```python
from build123d import *

# Parameters (mm, degrees)
BOSS_EXTRUDE1_DEPTH = 4
SKETCH2_W           = 92
SKETCH2_H           = 107
BOSS_EXTRUDE2_DEPTH = 13.5
SKETCH3_W           = 84
SKETCH3_H           = 27.9
BOSS_EXTRUDE3_DEPTH = 15
SKETCH4_W           = 79
SKETCH4_H           = 9
CUT_EXTRUDE1_DEPTH  = 89.324685111
SKETCH5_W           = 54
SKETCH5_H           = 8
CUT_EXTRUDE2_DEPTH  = 1
BOSS_EXTRUDE4_DEPTH = 17


with BuildPart() as part:
    # Sketch1 → Boss-Extrude1 (new body)
    with BuildSketch(Plane.XY):
        with BuildLine():
            Line((22.5, 58.5), (22.5, 67))
            Line((22.5, 67), (-22.5, 67))
            Line((-22.5, 67), (-22.5, 58.5))
            ThreePointArc((-22.5, 58.5), (-25.5, 55.5), (-28.5, 58.5))
            Line((-28.5, 58.5), (-28.5, 67))
            Line((-28.5, 67), (-50, 67))
            Line((-50, 67), (-50, 61.5))
            Line((-50, 61.5), (-42, 61.5))
            ThreePointArc((-42, 61.5), (-39, 58.5), (-42, 55.5))
            Line((-42, 55.5), (-50, 55.5))
            Line((-50, 55.5), (-50, -55.5))
            Line((-50, -55.5), (-42, -55.5))
            ThreePointArc((-42, -55.5), (-39, -58.5), (-42, -61.5))
            Line((-42, -61.5), (-50, -61.5))
            Line((-50, -61.5), (-50, -67))
            Line((-50, -67), (-28.5, -67))
            Line((-28.5, -67), (-28.5, -58.5))
            ThreePointArc((-28.5, -58.5), (-25.5, -55.5), (-22.5, -58.5))
            Line((-22.5, -58.5), (-22.5, -67))
            Line((-22.5, -67), (22.5, -67))
            Line((22.5, -67), (22.5, -58.5))
            ThreePointArc((22.5, -58.5), (25.5, -55.5), (28.5, -58.5))
            Line((28.5, -58.5), (28.5, -67))
            Line((28.5, -67), (50, -67))
            Line((50, -67), (50, -61.5))
            Line((50, -61.5), (42, -61.5))
            ThreePointArc((42, -61.5), (39, -58.5), (42, -55.5))
            Line((42, -55.5), (50, -55.5))
            Line((50, -55.5), (50, 55.5))
            Line((50, 55.5), (42, 55.5))
            ThreePointArc((42, 55.5), (39, 58.5), (42, 61.5))
            Line((42, 61.5), (50, 61.5))
            Line((50, 61.5), (50, 67))
            Line((50, 67), (28.5, 67))
            Line((28.5, 67), (28.5, 58.5))
            ThreePointArc((28.5, 58.5), (25.5, 55.5), (22.5, 58.5))
        make_face()
    extrude(amount=BOSS_EXTRUDE1_DEPTH)

    # Sketch2 → Boss-Extrude2 (add)
    with BuildSketch(Plane.XY):
        Rectangle(SKETCH2_W, SKETCH2_H)
    extrude(amount=BOSS_EXTRUDE2_DEPTH)

    # Sketch3 → Boss-Extrude3 (add)
    with BuildSketch(Plane.XY.offset(13.5)):
        Rectangle(SKETCH3_W, SKETCH3_H)
    extrude(amount=BOSS_EXTRUDE3_DEPTH)

    # Sketch4 → Cut-Extrude1 (cut, through all)
    with BuildSketch(Plane.XY.offset(28.5)):
        with Locations((0, 7.45)):
            Rectangle(SKETCH4_W, SKETCH4_H)
    extrude(amount=-CUT_EXTRUDE1_DEPTH, mode=Mode.SUBTRACT)

    # Sketch5 → Cut-Extrude2 (cut)
    with BuildSketch(Plane.XY.offset(28.5)):
        with Locations((-0.051701633, -6.019148753)):
            Rectangle(SKETCH5_W, SKETCH5_H)
    extrude(amount=-CUT_EXTRUDE2_DEPTH, mode=Mode.SUBTRACT)

    # Sketch6 → Boss-Extrude4 (add)
    with BuildSketch(Plane(origin=(0, 0, 0), x_dir=(-1, 0, 0), z_dir=(0, 0, -1))):
        Polygon((-45, -53), (45, -53), (45, -3), (42, -3), (42, -50), (-42, -50), (-42, -3), (-45, -3), align=None)
    extrude(amount=BOSS_EXTRUDE4_DEPTH)


solid = part.part
```
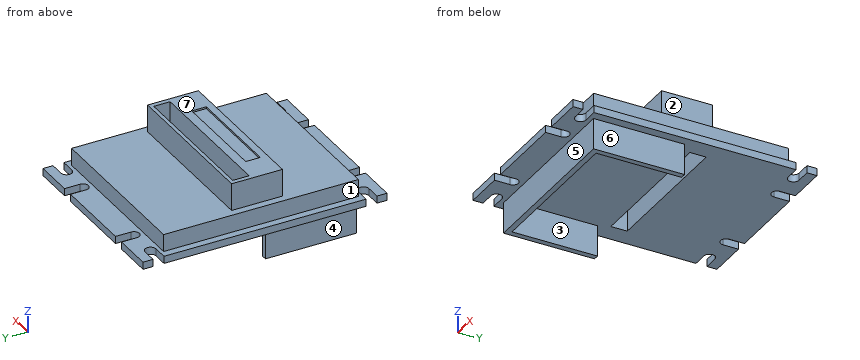
Check sheet for the modelled part. Datum: model origin and axes. Units: mm. Face numbers are marked on the shaded views. A direction names the side the tool comes from. Round coordinates to 2 decimals unless told otherwise and drop trailing zeros. Write each loop counter-clockwise with the first axis right and the second up, starting at its lowest first coordinate (ties: lowest second). Pieces come first, ordered by that corner, then holes. Notation, with made-up numbers: (74, -39.75) -> (129, -39.75) arc R13 cw to (129, -15.75) -> close; hole circle Ø7 at (68.5, 63.25). An arc over 180 degrees is marked (long way). Put each result on its own line as item: value.
(1) Sectioned sample at A-A (z = 5.5). Enter the section's corners in (x, y), plus the area to 3 significant figures.
Values found:
outline: (-46, -53.5) -> (46, -53.5) -> (46, 53.5) -> (-46, 53.5) -> close; hole (-39.5, 2.95) -> (39.5, 2.95) -> (39.5, 11.95) -> (-39.5, 11.95) -> close
area: 9,130 mm^2
(2) Sectioned sample at C-C (y = 18.5). Enter the section's corners in (x, z), plus the area to 3 significant figures.
Values found:
outline: (-50, 0) -> (50, 0) -> (50, 4) -> (46, 4) -> (46, 13.5) -> (-46, 13.5) -> (-46, 4) -> (-50, 4) -> close
area: 1,270 mm^2
(3) Tool access check on the marked faces 1, 2, 3, 4 and 5. Record the directions out of +Z, -Z, +X, -X, +Y, -Y that give a thin tool (end or side, any length) a straight path to the whole face; none if there is none.
Values found:
face 1: +Z, -X, +Y, -Y
face 2: +Z, +X, +Y, -Y
face 3: -Z, +Y
face 4: -Z, -X, +Y, -Y
face 5: -Z, +X, -X, -Y
(4) Sectioned sample at D-D (z = -14). Enter the section's corners in (x, y).
Values found:
outline: (-45, -53) -> (45, -53) -> (45, -3) -> (42, -3) -> (42, -50) -> (-42, -50) -> (-42, -3) -> (-45, -3) -> close
(5) Sectioned sample at B-B (x = 25.5). Enter the section's corners in (y, z).
Values found:
outline: (-55.5, 0) -> (-53, 0) -> (-53, -17) -> (-50, -17) -> (-50, 0) -> (2.95, 0) -> (2.95, 28.5) -> (-2.02, 28.5) -> (-2.02, 27.5) -> (-10.02, 27.5) -> (-10.02, 28.5) -> (-13.95, 28.5) -> (-13.95, 13.5) -> (-53.5, 13.5) -> (-53.5, 4) -> (-55.5, 4) -> close; (11.95, 0) -> (55.5, 0) -> (55.5, 4) -> (53.5, 4) -> (53.5, 13.5) -> (13.95, 13.5) -> (13.95, 28.5) -> (11.95, 28.5) -> close
(6) Go/stop test with flat-tipped pins: pin 1 Ø7 at (y, z) = (8, 19) entering from -X; pin 2 Ø5 at (y, z) = (23.5, 7) entering from -X; pin 3 Ø5 at (y, z) = (-34.5, -12) entering from +X. Record where each tip stops, or that it passes through.
Values found:
pin 1: stops at x = -42
pin 2: stops at x = -46
pin 3: stops at x = 45
(7) Mould release check, pull along Z, two halves, no side actions. Record for the marked faces 6 and 7: released by +Z, released by -Z, zero draft, split by the parting line, or undercut.
Values found:
face 6: zero draft
face 7: released by +Z
(8) Material ranges on line 1 (Y direction, x = -28.5, z = 10); line 2 (X direction, y = 11, z = 10); line 3 (Y direction, x = -30.5, z = 1), recorded low to high.
Values found:
line 1: y = -53.5 to 2.95, 11.95 to 53.5
line 2: x = -46 to -39.5, 39.5 to 46
line 3: y = -67 to 2.95, 11.95 to 67
